```python
from build123d import *

# Parameters (mm, degrees)
EXTRUDE_THIN1_DEPTH      = 6.35
EXTRUDE_THIN1_DEPTH_BACK = 6.35
CUT_EXTRUDE2_DEPTH       = 57.058652321
CUT_EXTRUDE2_DEPTH_BACK  = 57.058652321
SKETCH2_R                = 2.8


with BuildPart() as part:
    # Sketch1 → Extrude-Thin1 (new, two sides: drawn at the far end of the back side and taken through both)
    with BuildSketch(Plane.XY.offset(-EXTRUDE_THIN1_DEPTH_BACK)):
        Polygon((-42.5, 0), (-16.5, 0), (-16.5, 33), (16.5, 33), (16.5, 0), (42.5, 0), (42.5, 3), (19.5, 3), (19.5, 36), (-19.5, 36), (-19.5, 3), (-42.5, 3), align=None)
    extrude(amount=EXTRUDE_THIN1_DEPTH + EXTRUDE_THIN1_DEPTH_BACK)

    # Sketch2 → Cut-Extrude2 (cut, two sides: drawn at the far end of the back side and taken through both)
    with BuildSketch(Plane(origin=(0, 0, 0), x_dir=(1, 0, 0), z_dir=(0, 1, 0)).offset(-CUT_EXTRUDE2_DEPTH_BACK)):
        with Locations(Location((32.5, 0, 0), (0, 0, 270))):
            Circle(SKETCH2_R)
        with Locations(Location((-32.5, 0, 0), (0, 0, 270))):
            Circle(SKETCH2_R)
    extrude(amount=CUT_EXTRUDE2_DEPTH + CUT_EXTRUDE2_DEPTH_BACK, mode=Mode.SUBTRACT)


solid = part.part
```
Design review of the part built by this model. Coordinates are the model's own, in mm. A direction names the side the tool comes from. Give positions to 0.01 mm unless a question says otherwise; leave off trailing zeros. Order: outer loops, then holes, each group sorted by start corner. A loop starts at its lowest first (then second) coordinate and runs counter-clockwise, first axis right, second up. Notation, with made-up numbers: M -18.5,-17 L 2.5,-17 A34 cw 2.5,15 Z; hole C 19.25,64.25 d2. An arc over 180 degrees is marked long. One line per question, with ' | ' between items. Start each with the question number.
Q1. The part is to be moulded in two halves that separate along X. For faces 6 (the face through (-3, 34, -6.35)), 7 (the face through (19.5, 19, 0)), 8 (the face through (-42.5, 2, 0)), 9 (the face through (0, 33, 0)), say which applies: +X half, -X half, draft (parallel to the pull), parting line (faces both ways), or undercut.
Q2. For L1, parallel to X at y = 1.1, z = 0; L2, parallel to X at y = 8.5, z = -5.25; L3, parallel to Z at x = -32.5, y = 1.45, list the stretches that pass through material, from the lowest coordinate up. Write a range as [from, to].
Q3. For pin 1 Ø2 at (x, z) = (-6.5, 1.5) entering from -Y; pin 2 Ø4 at (y, z) = (22.5, 2.5) entering from -X; pin 3 Ø4 at (y, z) = (9, 0.5) entering from +X, all flat-tipped, find the tip position at first contact; note any pin that passes through.
Q4. We need section D-D (y = 34.5). Write out the cut boundary in (x, z), plus the area to 3 significant figures.
Q5. We need section C-C (z = 0). Write out the cut boundary in (x, y), plus the area to 3 significant figures.
Q6. Machinability: for faces 1 (the face through (-16.5, 16, 0)), 2 (the face through (-3, 34, 6.35)), 3 (the face through (-28, 3, 0)), 4 (the face through (29, 3, 0)), 5 (the face through (42.5, 1, 0)), which of the approach directions +Z, -Z, +X, -X, +Y, -Y give a long, thin tool a straight path to every point of the face, cutting with its end or side? Answer none if there is none.
Q7. We need section A-A (y = 20.5). Write out the cut boundary in (x, z), plus the area to 3 significant figures.
Q8. We need section B-B (x = -32.5). Write out the cut boundary in (y, z), plus the area to 3 significant figures.
Returned:
1) face 6: draft | face 7: +X half | face 8: -X half | face 9: undercut
2) L1: [-42.5, -35.3], [-29.7, -16.5], [16.5, 29.7], [35.3, 42.5] | L2: [-19.5, -16.5], [16.5, 19.5] | L3: [-6.35, -2.8], [2.8, 6.35]
3) pin 1: y = 33 | pin 2: x = -19.5 | pin 3: x = 19.5
4) outline: M -19.5,-6.35 L 19.5,-6.35 L 19.5,6.35 L -19.5,6.35 Z | area: 495 mm2
5) outline: M -42.5,0 L -35.3,0 L -35.3,3 L -42.5,3 Z; M -29.7,0 L -16.5,0 L -16.5,33 L 16.5,33 L 16.5,0 L 29.7,0 L 29.7,3 L 19.5,3 L 19.5,36 L -19.5,36 L -19.5,3 L -29.7,3 Z; M 35.3,0 L 42.5,0 L 42.5,3 L 35.3,3 Z | area: 419 mm2
6) face 1: +Z, -Z, -Y | face 2: +Z, +X, -X, +Y, -Y | face 3: +Z, -Z, -X, +Y | face 4: +Z, -Z, +X, +Y | face 5: +Z, -Z, +X, +Y, -Y
7) outline: M -19.5,-6.35 L -16.5,-6.35 L -16.5,6.35 L -19.5,6.35 Z; M 16.5,-6.35 L 19.5,-6.35 L 19.5,6.35 L 16.5,6.35 Z | area: 76.2 mm2
8) outline: M 0,-6.35 L 3,-6.35 L 3,-2.8 L 0,-2.8 Z; M 0,2.8 L 3,2.8 L 3,6.35 L 0,6.35 Z | area: 21.3 mm2
